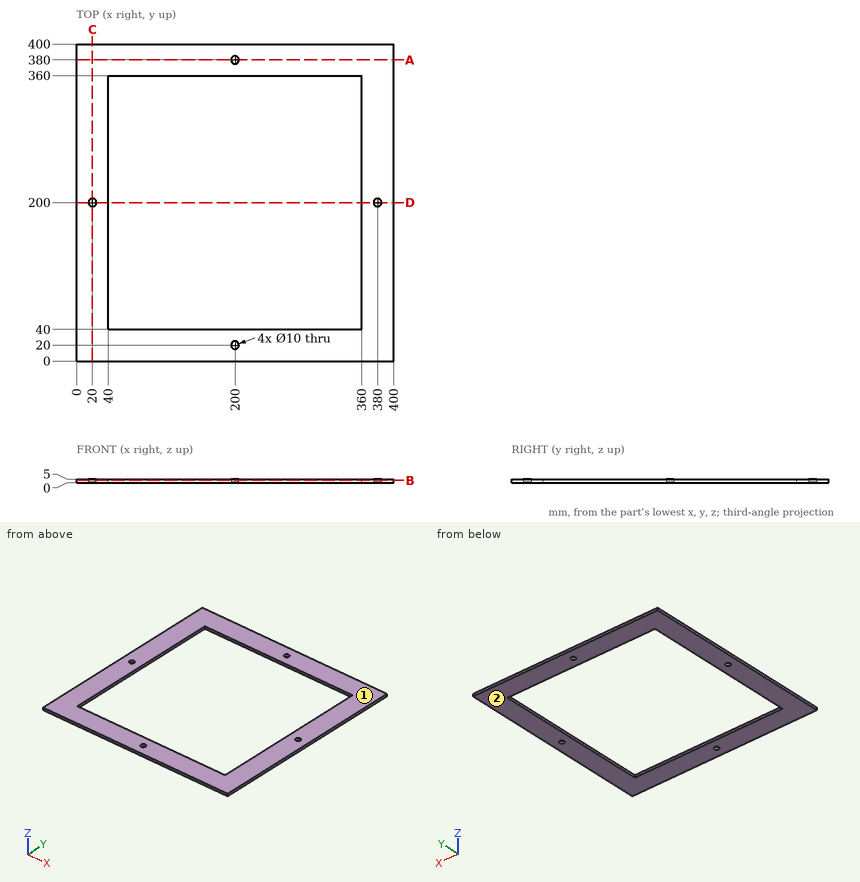
Answer from the drawing. Dimensions are ordinates in mm from the lowest x, y and z of the part. Round coordinates to 2 decimals unless told otherwise and drop trailing zeros. Loops run counter-clockwise (first coordinate to the right, second up) from the corner with the lowest first, then second, coordinate; pieces in that order, holes last.
1) For a pull along Z with two mould halves and no side action, classify the marked faces 1 and 2 as released by +Z, released by -Z, zero draft, split by the parting line, or undercut.
Outcome:
face 1: released by +Z
face 2: released by -Z
2) A cutting plane is placed at A-A on y = 380. Determine the outline of the cut face in (x, z), plus the area to 3 significant figures.
Outcome:
outline: (0, 0) - (195, 0) - (195, 5) - (0, 5) - close; (205, 0) - (400, 0) - (400, 5) - (205, 5) - close
area: 1,950 mm2
3) A cutting plane is placed at D-D on y = 200. Determine the outline of the cut face in (x, z).
Outcome:
outline: (0, 0) - (15, 0) - (15, 5) - (0, 5) - close; (25, 0) - (40, 0) - (40, 5) - (25, 5) - close; (360, 0) - (375, 0) - (375, 5) - (360, 5) - close; (385, 0) - (400, 0) - (400, 5) - (385, 5) - close
4) Consider line 1 (Y direction, x = 200, z = 3.45); line 2 (Y direction, x = 380, z = 3.35). Determine where each line is inside the solid, lowest interval first.
Outcome:
line 1: y = 0 to 15, 25 to 40, 360 to 375, 385 to 400
line 2: y = 0 to 195, 205 to 400
5) A cutting plane is placed at B-B on z = 3.2. Determine the outline of the cut face in (x, y), plus the area to 3 significant figures.
Outcome:
outline: (0, 0) - (400, 0) - (400, 400) - (0, 400) - close; hole circle Ø10 at (20, 200); hole (40, 40) - (360, 40) - (360, 360) - (40, 360) - close; hole circle Ø10 at (200, 20); hole circle Ø10 at (200, 380); hole circle Ø10 at (380, 200)
area: 57,300 mm2
